The model under review builds one solid part; all positions refer to its coordinate system, in mm. Round coordinates to 2 decimals unless told otherwise and drop trailing zeros. Order: outer loops, then holes, each group sorted by start corner. A loop starts at its lowest first (then second) coordinate and runs counter-clockwise, first axis right, second up. Notation, with made-up numbers: M -4.5,83.25 L 32.5,83.25 A14 cw 32.5,106.25 Z; hole C 84,16 d10. An arc over 180 degrees is marked long. Answer as a JSON object with one key per item and string values. Group by question number.
1) The part is to be moulded in two halves that separate along X. For faces 1 (the cylindrical face through (-0.108, 9.949, 0.488)), 2 (the cylindrical face through (-0.108, 0.544, 0.488)), say which applies: +X half, -X half, draft (parallel to the pull), parting line (faces both ways), or undercut.
2) Consider section B-B, the plane z = 0. Write out the cut boundary in (x, y), then the cut area to 3 significant figures.
3) Consider section D-D, the plane x = 3.5. Write out the cut boundary in (y, z), then the cut area to 3 significant figures.
4) To check wall thickness, follow line 1 (Z direction, x = 0, y = 6.5); line 2 (Y direction, x = -1.5, z = -2); line 3 (X direction, y = 18.75, z = -0.25). State the ranges of each line that lie inside material, in increasing order.
5) Consider section C-C, the plane y = 17.5. Write out the cut boundary in (x, z).
6) Insertion check: pin 1 Ø3 at (x, z) = (-1, -2) entering from +Y; pin 2 Ø2 at (x, y) = (3, 6.5) entering from -Z; pin 3 Ø1 at (x, z) = (-2, 3) entering from -Y; pin 4 Ø2 at (x, z) = (-1.5, 3.5) entering from +Y. Each pin has a flat end and moves straight along its axis. Give the tip position at first contact, or say it passes through.
7) Consider section A-A, the plane x = 0. Write out the cut boundary in (y, z).
```python
from build123d import *

# Parameters (mm, degrees)
SKETCH_1_R               = 0.5
EXTRUDE_1_DEPTH          = 19.15
SKETCH_2_R               = 1.75
SKETCH_2_R_2             = 0.5
EXTRUDE_2_DEPTH          = 0.1
EXTRUDE_3_DEPTH          = 0.5
PATTERN_CIRCULAR_1_COUNT = 3
FILLET_2_R               = 0.3
FILLET_3_R               = 0.1


with BuildPart() as part:
    # Эскиз1 → Бобышка-Вытянуть1 (new body)
    with BuildSketch(Plane(origin=(0, 0, 0), x_dir=(1, 0, 0), z_dir=(0, 1, 0))):
        Circle(SKETCH_1_R)
    extrude(amount=EXTRUDE_1_DEPTH)

    # Эскиз2 → Бобышка-Вытянуть2 (add)
    with BuildSketch(Plane(origin=(0, 1, 0), x_dir=(1, 0, 0), z_dir=(0, 1, 0))):
        Circle(SKETCH_2_R)
        Circle(SKETCH_2_R_2, mode=Mode.SUBTRACT)
    extrude(amount=EXTRUDE_2_DEPTH)

    # Эскиз3 → Бобышка-Вытянуть3 (add, symmetric)
    with BuildSketch(Plane.XY):
        Polygon((1.5, 1), (2.303369234, 1), (2.639009087, 0.6), (5, 0.6), (5, 0.7), (2.685639852, 0.7), (2.35, 1.1), (1.5, 1.1), align=None)
    extrude_3 = extrude(amount=EXTRUDE_3_DEPTH, both=True)

    # Круговой массив1: Бобышка-Вытянуть3 ×3 about axis
    pattern_circular_1_axis = Axis((0, 0, 0), (0, 1, 0))
    for i in range(1, PATTERN_CIRCULAR_1_COUNT):
        add(extrude_3.rotate(pattern_circular_1_axis, i * 360 / PATTERN_CIRCULAR_1_COUNT))

    # Скругление2
    fillet_2_edges = [part.edges().sort_by_distance(p)[0] for p in [
        (2.303369234, 1, 0),
        (2.639009087, 0.6, 0),
        (2.685639852, 0.7, 0),
        (2.35, 1.1, 0),
        (-1.151684617, 1, -1.994776271),
        (-1.319504543, 0.6, -2.28544891),
        (-1.342819926, 0.7, -2.325832338),
        (-1.175, 1.1, -2.035159699),
        (-1.151684617, 1, 1.994776271),
        (-1.319504543, 0.6, 2.28544891),
        (-1.342819926, 0.7, 2.325832338),
        (-1.175, 1.1, 2.035159699),
    ]]
    fillet(fillet_2_edges, radius=FILLET_2_R)

    # Скругление3
    fillet_3_edges = [part.edges().sort_by_distance(p)[0] for p in [
        (-0.5, 0, 0),
        (-0.5, 19.15, 0),
    ]]
    fillet(fillet_3_edges, radius=FILLET_3_R)


solid = part.part
```
Results list:
{
 "1": {"face 1": "parting line", "face 2": "undercut"},
 "2": {"outline": "M -1.75,1 L -0.5,1 L -0.5,0.1 A0.1 ccw -0.4,0 L 0.4,0 A0.1 ccw 0.5,0.1 L 0.5,1 L 2.16,1 A0.3 cw 2.39,0.89 L 2.55,0.71 A0.3 ccw 2.78,0.6 L 5,0.6 L 5,0.7 L 2.83,0.7 A0.3 cw 2.6,0.81 L 2.44,0.99 A0.3 ccw 2.21,1.1 L 0.5,1.1 L 0.5,19.05 A0.1 ccw 0.4,19.15 L -0.4,19.15 A0.1 ccw -0.5,19.05 L -0.5,1.1 L -1.75,1.1 Z", "area": "19.7 mm^2"},
 "3": {"outline": "M 0.6,-0.5 L 0.7,-0.5 L 0.7,0.5 L 0.6,0.5 Z", "area": "0.100 mm^2"},
 "4": {"line 1": "-0.5 to 0.5", "line 2": "0.79 to 0.94", "line 3": "-0.43 to 0.43"},
 "5": {"outline": "C 0,0 d1"},
 "6": {"pin 1": "y = 1.1", "pin 2": "through", "pin 3": "y = 0.6", "pin 4": "y = 0.7"},
 "7": {"outline": "M 0,-0.4 A0.1 ccw 0.1,-0.5 L 1,-0.5 L 1,-1.75 L 1.1,-1.75 L 1.1,-0.5 L 19.05,-0.5 A0.1 ccw 19.15,-0.4 L 19.15,0.4 A0.1 ccw 19.05,0.5 L 1.1,0.5 L 1.1,1.75 L 1,1.75 L 1,0.5 L 0.1,0.5 A0.1 ccw 0,0.4 Z"}
}
